```python
from build123d import *

# Parameters (mm, degrees)
F1_DEPTH = 5
F2_DEPTH = 5


with BuildPart() as f1:
    # F0 (on Front) → F1 (new body)
    with BuildSketch(Plane.XZ):
        with BuildLine():
            ThreePointArc((11.124385, 0), (7.783139, 27.203268), (0, 53.482622))
            ThreePointArc((0, 53.482622), (-7.783139, 27.203268), (-11.124385, 0))
            Line((-11.124385, 0), (11.124385, 0))
        make_face()
    extrude(amount=F1_DEPTH)

    # F0 (on Front) → F2 (join)
    with BuildSketch(Plane.XZ):
        with BuildLine():
            Line((11.124385, 0), (-11.124385, 0))
            Line((-11.124385, 0), (-11.124385, -38.364865))
            Line((-11.124385, -38.364865), (-4.081059, -26.264793))
            ThreePointArc((-4.081059, -26.264793), (0.14515, -23.743036), (4.52543, -25.986524))
            Line((4.52543, -25.986524), (12.621719, -38.031906))
            Line((12.621719, -38.031906), (11.124385, 0))
        make_face()
    extrude(amount=F2_DEPTH)


solid = f1.part
```
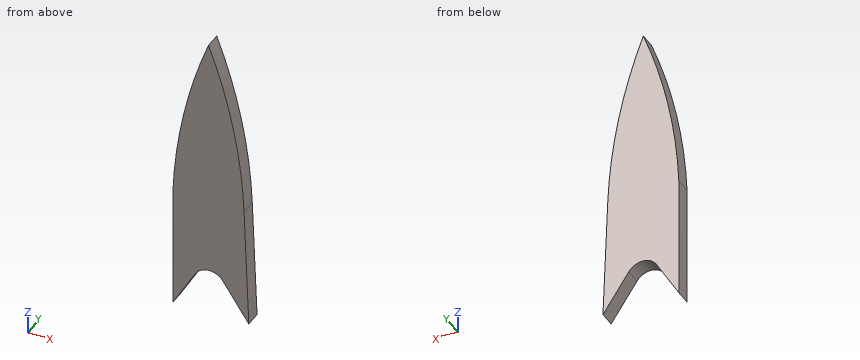
Work out the finished part from the listing and answer in its coordinate system (mm). Give positions to 0.01 mm unless a question says otherwise; leave off trailing zeros. Order: outer loops, then holes, each group sorted by start corner. A loop starts at its lowest first (then second) coordinate and runs counter-clockwise, first axis right, second up.
1. Section A-A, the plane y = -4.15 is taken. Determine the outline of the cut face in (x, z), and give its area (3 significant figures).
Result sheet:
outline: (-11.12, -38.36) - (-4.08, -26.26) arc R5.08 cw to (4.53, -25.99) - (12.62, -38.03) - (11.12, 0) arc R165.57 ccw to (0, 53.48) arc R165.57 ccw to (-11.12, 0) - close
area: 1,430 mm2
2. This flat-tipped pin is pushed along its axis until it touches: P1, Ø1, axis at y = -1.5, z = 38.5, coming from the +X side. Where does it stop, or does it pass through?
Result sheet:
P1: stops at x = 5.16
3. Section C-C, the plane x = 1.25 is taken. Determine the outline of the cut face in (y, z), and give its area (3 significant figures).
Result sheet:
outline: (-5, -23.83) - (0, -23.83) - (0, 50.16) - (-5, 50.16) - close
area: 370 mm2
4. Section B-B, the plane z = 22 is taken. Determine the outline of the cut face in (x, y), and give its area (3 significant figures).
Result sheet:
outline: (-8.78, -5) - (8.78, -5) - (8.78, 0) - (-8.78, 0) - close
area: 87.8 mm2
5. Straight lines are drawn through the part: L1, parallel to X at y = -3.5, z = 6; L2, parallel to X at y = -0.9, z = -17. For each, find the intervals that lie inside material, in ascending order.
Result sheet:
L1: x = -10.78 to 10.78
L2: x = -11.12 to 11.79
